Geometry check sheet. Reference: drawing and pictorial views, mm from the part's lowest x, y, z. Give positions to 0.01 mm unless a question says otherwise; leave off trailing zeros. Loops run counter-clockwise (first coordinate to the right, second up) from the corner with the lowest first, then second, coordinate; pieces in that order, holes last. Notation, with made-up numbers: M -22,75 L 10,75 A18 cw 10,92 Z; hole C -34,8.25 d3. An arc over 180 degrees is marked long. One line per question, with ' | ' between items. Start each with the question number.
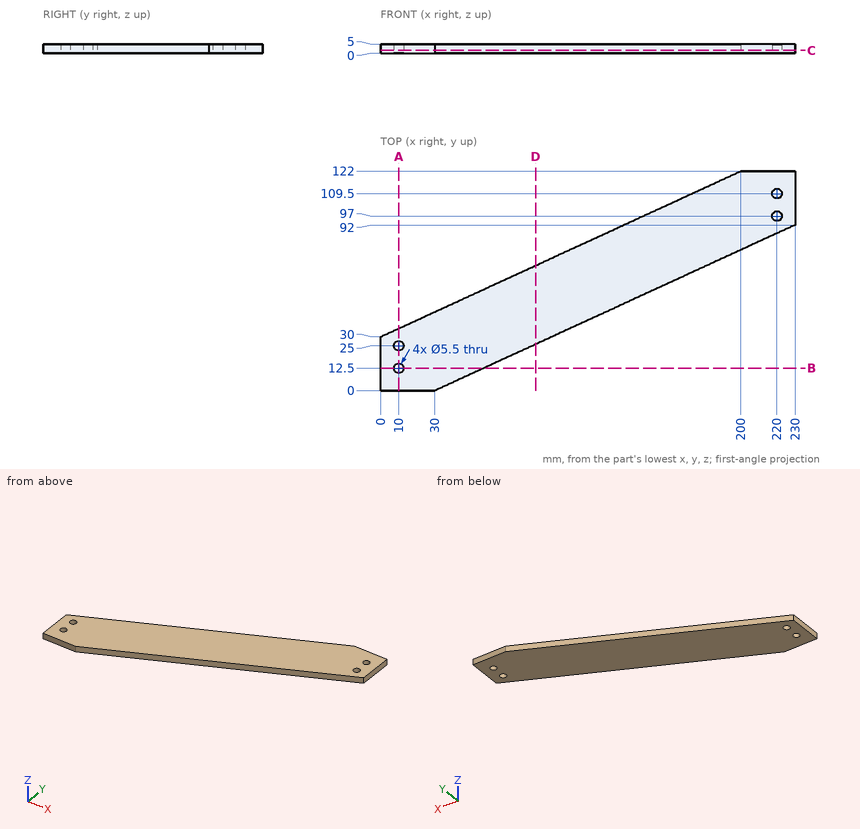
Q1. Cross-section at C-C (z = 1.4). Record the cut outline in (x, y).
Q2. Cross-section at D-D (x = 86). Record the cut outline in (y, z), and give its area (3 significant figures).
Q3. Depth check by flat-ended pin: P1, Ø1.5, axis at y = 92, z = 0.5, coming from the -X side. Enter the tip coordinate at first touch or a pass-through.
Q4. Cross-section at B-B (y = 12.5). Record the cut outline in (x, z).
Q5. Material ranges on probe 1 along Y at (x, z) = (10, 4.05); probe 2 along Y at (x, z) = (220, 1.55); probe 3 along X at (y, z) = (15.5, 0.2), recorded low to high. Write a range as from..to.
Q6. Cross-section at A-A (x = 10). Record the cut outline in (y, z), and give its area (3 significant figures).
Solved:
1) outline: M 0,0 L 30,0 L 230,92 L 230,122 L 200,122 L 0,30 Z; hole C 10,12.5 d5.5; hole C 10,25 d5.5; hole C 220,97 d5.5; hole C 220,109.5 d5.5
2) outline: M 25.76,0 L 69.56,0 L 69.56,5 L 25.76,5 Z | area: 219 mm²
3) P1: stops at x = 133.15
4) outline: M 0,0 L 7.25,0 L 7.25,5 L 0,5 Z; M 12.75,0 L 57.17,0 L 57.17,5 L 12.75,5 Z
5) probe 1: y = 0..9.75, 15.25..22.25, 27.75..34.6 | probe 2: y = 87.4..94.25, 99.75..106.75, 112.25..122 | probe 3: x = 0..63.7
6) outline: M 0,0 L 9.75,0 L 9.75,5 L 0,5 Z; M 15.25,0 L 22.25,0 L 22.25,5 L 15.25,5 Z; M 27.75,0 L 34.6,0 L 34.6,5 L 27.75,5 Z | area: 118 mm²
